Geometry check sheet. Reference: the model listing, model coordinates, mm. Face numbers are marked on the shaded views. Round coordinates to 2 decimals unless told otherwise and drop trailing zeros. Order: outer loops, then holes, each group sorted by start corner. A loop starts at its lowest first (then second) coordinate and runs counter-clockwise, first axis right, second up.
```python
from build123d import *

# Parameters (mm, degrees)
F0_W           = 60
F0_H           = 60
F1_DEPTH       = 10
F2_R           = 4
F3_DEPTH       = 10.001
F4_D           = 5.5
F4_CBORE_D     = 9.75
F4_CBORE_DEPTH = 5


with BuildPart() as f1:
    # F0 (on Top) → F1 (new body)
    with BuildSketch(Plane.XY):
        Rectangle(F0_W, F0_H)
    extrude(amount=-F1_DEPTH)

    # F2 (on face) → F3 (cut, through all)
    with BuildSketch(Plane.XY):
        with Locations((0, -21.2132034356)):
            Circle(F2_R)
        with Locations((-10.6066017178, -10.6066017178)):
            Circle(F2_R)
        with Locations((-21.2132034356, 0)):
            Circle(F2_R)
        Circle(F2_R)
        with Locations((10.6066017178, -10.6066017178)):
            Circle(F2_R)
        with Locations((21.2132034356, 0)):
            Circle(F2_R)
        with Locations((10.6066017178, 10.6066017178)):
            Circle(F2_R)
        with Locations((0, 21.2132034356)):
            Circle(F2_R)
        with Locations((-10.6066017178, 10.6066017178)):
            Circle(F2_R)
    extrude(amount=-F3_DEPTH, mode=Mode.SUBTRACT)

    # F4 (through all)
    with Locations(Plane.XY):
        with Locations((23, -23), (-23, -23), (-23, 23), (23, 23)):
            CounterBoreHole(F4_D / 2, F4_CBORE_D / 2, F4_CBORE_DEPTH)


solid = f1.part
```
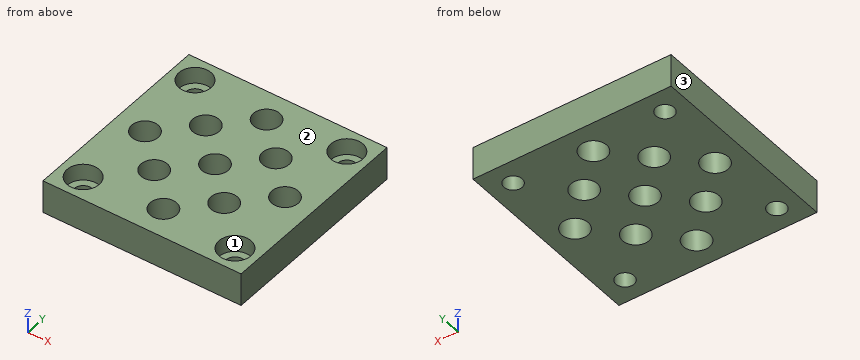
(1) Sectioned sample at C-C, the plane y = 13. Record the cut outline in (x, z), and give its area (3 significant figures).
Returned:
outline: (-30, -10) - (-13.81, -10) - (-13.81, 0) - (-30, 0) - close; (-7.4, -10) - (7.4, -10) - (7.4, 0) - (-7.4, 0) - close; (13.81, -10) - (30, -10) - (30, 0) - (13.81, 0) - close
area: 472 mm2
(2) Sectioned sample at B-B, the plane x = 1.5. Record the cut outline in (y, z), and give its area (3 significant figures).
Returned:
outline: (-30, -10) - (-24.92, -10) - (-24.92, 0) - (-30, 0) - close; (-17.51, -10) - (-3.71, -10) - (-3.71, 0) - (-17.51, 0) - close; (3.71, -10) - (17.51, -10) - (17.51, 0) - (3.71, 0) - close; (24.92, -10) - (30, -10) - (30, 0) - (24.92, 0) - close
area: 378 mm2
(3) Sectioned sample at A-A, the plane y = 0. Record the cut outline in (x, z), and give its area (3 significant figures).
Returned:
outline: (-30, -10) - (-25.21, -10) - (-25.21, 0) - (-30, 0) - close; (-17.21, -10) - (-4, -10) - (-4, 0) - (-17.21, 0) - close; (4, -10) - (17.21, -10) - (17.21, 0) - (4, 0) - close; (25.21, -10) - (30, -10) - (30, 0) - (25.21, 0) - close
area: 360 mm2
(4) Sectioned sample at D-D, the plane x = -10. Record the cut outline in (y, z).
Returned:
outline: (-30, -10) - (-14.56, -10) - (-14.56, 0) - (-30, 0) - close; (-6.65, -10) - (6.65, -10) - (6.65, 0) - (-6.65, 0) - close; (14.56, -10) - (30, -10) - (30, 0) - (14.56, 0) - close
(5) Material ranges on line 1 (Y direction, x = 0, z = -7); line 2 (X direction, y = 9.5, z = -1.5); line 3 (Y direction, x = 1.5, z = -1.25), recorded low to high.
Returned:
line 1: y = -30 to -25.21, -17.21 to -4, 4 to 17.21, 25.21 to 30
line 2: x = -30 to -14.45, -6.76 to 6.76, 14.45 to 30
line 3: y = -30 to -24.92, -17.51 to -3.71, 3.71 to 17.51, 24.92 to 30
(6) Draft check along X on the marked faces 1, 2 and 3. Enter one of: released by +X, released by -X, zero draft, split by the parting line, or undercut.
Returned:
face 1: undercut
face 2: zero draft
face 3: released by -X
(7) Depth check by flat-ended pin: P1, Ø5, axis at x = 0, y = -21.21, coming from the -Z side; P2, Ø10.5, axis at x = 0, y = 21.21, coming from the -Z side; P3, Ø9, axis at x = 23, y = -23, coming from the +Z side. Enter the tip coordinate at first touch or a pass-through.
Returned:
P1: passes through
P2: stops at z = -10
P3: stops at z = -5
